from build123d import *

# Parameters (mm, degrees)
F2_R = 6.096
F4_R = 1.27


# Not quite as in the source:
# - a fillet or chamfer that OpenCascade refuses, or shapes differently, is made with other operations: its cross-section is extruded or revolved along the edge and cut away or added


with BuildPart() as f1:
    # F0 (on Front) → F1 (revolve)
    with BuildSketch(Plane.XZ):
        Polygon((38.2069466584, 0), (38.2069466584, 8.7376), (-18.9430533416, 8.7376), (-18.9430533416, 3.9624), (-25.2930533416, 3.9624), (-25.2930533416, 0), align=None)
    revolve(axis=Axis((6.4569466584, 0, 0), (-1, 0, 0)))

    # F2
    f2_edges = [f1.edges().sort_by_distance(p)[0] for p in [
        (38.206947, 0, -8.7376),
    ]]
    fillet(f2_edges, radius=F2_R)

    # F3: fillet of radius 7.62 on 1 edges, made by hand

    # F3_s1 → F3_t2 (revolve, cut)
    with BuildSketch(Plane.XZ):
        with BuildLine():
            ThreePointArc((-11.8740001546, 8.7376), (-16.139385483, 7.4319398705), (-18.9430533416, 3.9624))
            Line((-18.9430533416, 3.9624), (-18.9430533416, 8.7376))
            Line((-18.9430533416, 8.7376), (-11.8740001546, 8.7376))
        make_face()
    revolve(axis=Axis((-18.9430533416, 0, 0), (-1, 0, 0)), mode=Mode.SUBTRACT)

    # F4
    f4_edges = [f1.edges().sort_by_distance(p)[0] for p in [
        (-25.293053, 0, -3.9624),
    ]]
    fillet(f4_edges, radius=F4_R)


solid = f1.part
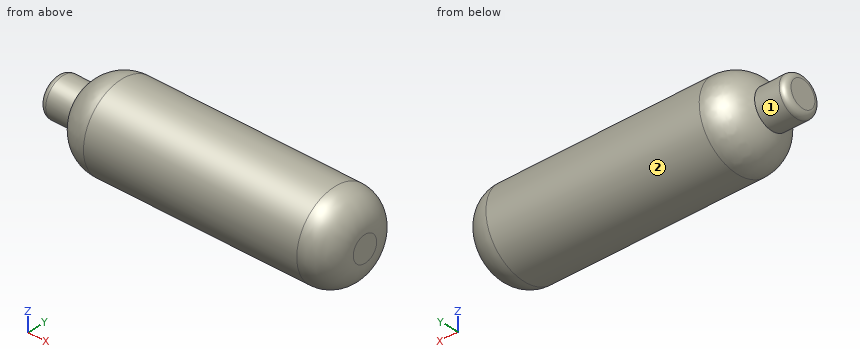
The listing builds one solid part. Answer for the finished solid, in the listing's coordinates (mm). Face numbers are marked on the shaded views. A direction names the side the tool comes from. Round coordinates to 2 decimals unless told otherwise and drop trailing zeros. Order: outer loops, then holes, each group sorted by start corner. A loop starts at its lowest first (then second) coordinate and runs counter-clockwise, first axis right, second up. Notation, with made-up numbers: (1.25, 25) -> (27.25, 25) arc R30 cw to (27.25, 49) -> close; hole circle Ø3 at (84, -17.5). An arc over 180 degrees is marked (long way). Put each result on its own line as item: value.
Q1. Section A-A, the plane x = 0.5 is taken. Write down the section's boundary in (y, z).
Results list:
outline: circle Ø17.48 at (0, 0)
Q2. Each of these flat-tipped pins is pushed along its axis until it touches: P1, Ø5, axis at x = 31, y = -4, coming from the -Z side; P2, Ø4, axis at y = 7, z = -6.5, coming from the -X side; P3, Ø3, axis at x = 24, z = 4.5, coming from the -Y side. Where does it stop, or does it pass through?
Results list:
P1: z = -8.61
P2: x = -15.96
P3: y = -8.21
Q3. Which of the six approach directions +Z, -Z, +X, -X, +Y, -Y give full straight-line access (tool end or side, diameter ignored) to the marked faces 1 and 2?
Results list:
face 1: -X
face 2: +X, -X
Q4. Consider line 1 along Z through (x, y) = (0.5, 0.25); line 2 along Z through (x, y) = (-2, -6.75); line 3 along X through (y, z) = (4.5, -5). Determine where each line is inside the solid, lowest interval first.
Results list:
line 1: -8.73 to 8.73
line 2: -5.55 to 5.55
line 3: -17.03 to 36.64
